Here's how the part is built. I have some questions about the finished solid (model axes, mm). Coordinates: 2 decimals unless noted, no trailing zeros. Order: outer loops, then holes, each group sorted by start corner. A loop starts at its lowest first (then second) coordinate and runs counter-clockwise, first axis right, second up. Notation, with made-up numbers: (-13, 7) - (2, 7) arc R27 ccw to (2, 44) - close; hole circle Ø11 at (1, 83.5). An arc over 180 degrees is marked (long way). Answer as CSV lines item,"result". Start each with the question number.
Item 1: Imagine slicing it at B-B on x = 24. List the corners of the cut face in (y, z) for me, and give its area (3 significant figures).
Item 2: I'm going to push flat-ended pins straight in: pin 1 (2 mm diameter, centred on x = 26.5, z = -16.5, fed in from +Y); pin 2 (3 mm diameter, centred on x = 7.5, z = -4.5, fed in from -Y); pin 3 (12 mm diameter, centred on x = 10.5, z = -21.5, fed in from +Y). Where does each tip first touch, or does it pass through?
Item 3: Imagine slicing it at A-A on z = -19.5. List the corners of the cut face in (x, y) for me, and give its area (3 significant figures).
Item 4: I need wall thicknesses on line 1 (Y direction, x = 39.5, z = -13.75); line 2 (Y direction, x = 29, z = -20.75). Which ranges of each line are inside material? Lowest first, please.
from build123d import *

# Parameters (mm, degrees)
SKETCH1_W           = 25.4
SKETCH1_H           = 682.499465201
BOSS_EXTRUDE1_DEPTH = 44.45
CUT_EXTRUDE1_DEPTH  = 44.45
CUT_EXTRUDE2_DEPTH  = 44.45


with BuildPart() as part:
    # Sketch1 → Boss-Extrude1 (new body)
    with BuildSketch(Plane(origin=(0, 0, 0), x_dir=(0, 0, -1), z_dir=(1, 0, 0))):
        with Locations((12.7, 341.249732601)):
            Rectangle(SKETCH1_W, SKETCH1_H)
    extrude(amount=BOSS_EXTRUDE1_DEPTH)

    # Sketch2 → Cut-Extrude1 (cut)
    with BuildSketch(Plane.XY):
        Polygon((44.45, 0), (0, 44.45), (0, 0), align=None)
    extrude(amount=-CUT_EXTRUDE1_DEPTH, mode=Mode.SUBTRACT)

    # Sketch3 → Cut-Extrude2 (cut)
    with BuildSketch(Plane.XY):
        Polygon((0, 638.049465201), (44.45, 682.499465201), (0, 682.499465201), align=None)
    extrude(amount=-CUT_EXTRUDE2_DEPTH, mode=Mode.SUBTRACT)


solid = part.part
Responses:
1,outline,"(20.45, -25.4) - (662.05, -25.4) - (662.05, 0) - (20.45, 0) - close"
1,area,"16,300 mm^2"
2,pin 1,"stops at y = 665.55"
2,pin 2,"stops at y = 35.45"
2,pin 3,"stops at y = 654.55"
3,outline,"(0, 44.45) - (44.45, 0) - (44.45, 682.5) - (0, 638.05) - close"
3,area,"28,400 mm^2"
4,line 1,"y = 4.95 to 677.55"
4,line 2,"y = 15.45 to 667.05"
